Autodesk Inventor part; units mm, degrees
ref_plane "Плоскость YZ" through (0, 0, 0) normal (1, 0, 0) x (0, 1, 0)
ref_plane "Плоскость XZ" through (0, 0, 0) normal (0, 1, 0) x (-1, 0, 0)
ref_plane "Плоскость XY" through (0, 0, 0) normal (0, 0, 1) x (1, 0, 0)
sketch "Эскиз1" plane through (0, 0, 0) normal (0, 1, 0) x (-1, 0, 0)
  line L0 (9.1667, 12.5) -> (-9.1667, 12.5)
  line L1 (-9.1667, 12.5) -> (-9.1667, -12.5)
  line L2 (-9.1667, -12.5) -> (9.1667, -12.5)
  line L3 (9.1667, -12.5) -> (9.1667, 12.5)
  line L4 (9.1667, 12.5) -> (-9.1667, -12.5) construction
  line L5 (-9.1667, 12.5) -> (9.1667, -12.5) construction
  line L6 (10.7667, 14.5) -> (-10.7667, 14.5)
  line L7 (-10.7667, 14.5) -> (-10.7667, -14.5)
  line L8 (-10.7667, -14.5) -> (10.7667, -14.5)
  line L9 (10.7667, -14.5) -> (10.7667, 14.5)
  line L10 (10.7667, 14.5) -> (-10.7667, -14.5) construction
  line L11 (-10.7667, 14.5) -> (10.7667, -14.5) construction
  circle A0 centre (6.6667, 10) radius 1.5
  circle A1 centre (6.6667, 3.3333) radius 1.5
  circle A2 centre (6.6667, -3.3333) radius 1.5
  circle A3 centre (6.6667, -10) radius 1.5
  circle A4 centre (0, 10) radius 1.5
  circle A5 centre (0, 3.3333) radius 1.5
  circle A6 centre (0, -3.3333) radius 1.5
  circle A7 centre (0, -10) radius 1.5
  circle A8 centre (-6.6667, 10) radius 1.5
  circle A9 centre (-6.6667, 3.3333) radius 1.5
  circle A10 centre (-6.6667, -3.3333) radius 1.5
  circle A11 centre (-6.6667, -10) radius 1.5
  point P0 (0, 0)
  dimension "d0" = 18.3333
  dimension "d1" = 25
  dimension "d2" = 1.6
  dimension "d3" = 2
  dimension "d4" = 3
  dimension "d5" = 2.5
  dimension "d6" = 2.5
  dimension "d9" = 6.6667
  dimension "d12" = 6.6667
extrude "Выдавливание1" add sketch "Эскиз1" along normal blind 1.8 contours L3 L2 L1 L0 | L9 L8 L7 L6
sketch "Эскиз2" plane through (0, 1.8, 0) normal (0, 1, 0) x (1, 0, 0)
  circle A0 centre (6.6667, 10) radius 1.5
  circle A1 centre (6.6667, -3.3333) radius 1.5
  circle A2 centre (0, 10) radius 1.5
  circle A3 centre (0, 3.3333) radius 1.5
  circle A4 centre (0, -3.3333) radius 1.5
  circle A5 centre (0, -10) radius 1.5
  circle A6 centre (-6.6667, 10) radius 1.5
  circle A7 centre (-6.6667, 3.3333) radius 1.5
  circle A8 centre (-6.6667, -3.3333) radius 1.5
  circle A9 centre (-6.6667, -10) radius 1.5
  circle A10 centre (6.6667, -10) radius 1.5
  circle A11 centre (6.6667, 3.3333) radius 1.5
  circle A12 centre (6.6667, 10) radius 1.5
  circle A13 centre (6.6667, 10) radius 2.8
  point P0 (0, 0)
  dimension "d39" = 5.6
extrude "Выдавливание2" cut sketch "Эскиз2" against normal blind 0.7 contours A13
sketch "Эскиз3" plane through (0, 1.8, 0) normal (0, 1, 0) x (1, 0, 0)
  line L0 (-10.7667, 14.5) -> (-10.7667, -14.5)
  line L1 (10.7667, 14.5) -> (-10.7667, 14.5)
  line L2 (-10.7667, -14.5) -> (-9.9667, -14.5)
  line L3 (-9.9667, -14.5) -> (-9.9667, 14.5)
  line L4 (-9.9667, 14.5) -> (-10.7667, 14.5)
  line L5 (-10.7667, 14.5) -> (-10.7667, -14.5)
  line L6 (10.7667, -14.5) -> (10.7667, 14.5)
  line L7 (10.7667, -14.5) -> (9.9667, -14.5)
  line L8 (9.9667, -14.5) -> (9.9667, 14.5)
  line L9 (9.9667, 14.5) -> (10.7667, 14.5)
  line L10 (10.7667, 14.5) -> (10.7667, -14.5)
  point P0 (0, 0)
  point P1 (9.9667, 14.5)
  dimension "d29" = 0.8
  dimension "d30" = 0.8
extrude "Выдавливание3" add sketch "Эскиз3" along normal blind 1.2
pattern_linear "Прямоуг.массив2" count 4 spacing 6.6667 along (0, 0, 1) count 3 spacing 6.6667 along (-1, 0, 0) of "Выдавливание2"
equation "\"d6\" = d5"
equation "\"d30\" = d29"
properties part number "HolesHelper" material "Типовой"
Design review of the part built by this model. Coordinates are the model's own, in mm. A direction names the side the tool comes from. Coordinates: 2 decimals unless noted, no trailing zeros. Order: outer loops, then holes, each group sorted by start corner. A loop starts at its lowest first (then second) coordinate and runs counter-clockwise, first axis right, second up. Notation, with made-up numbers: M 41,-14.5 L 67,-14.5 A11 ccw 67,-10.5 Z; hole C 31.25,51.25 d11. An arc over 180 degrees is marked long. Use a Markdown table: item, result.
(1) Add section B-B (z = -10). Count the separate pieces of the cut face and the enclosed holes in it, then the cut area to 3 significant figures.
Worked answers:
| item | result |
|---|---|
| separate pieces | 4 |
| enclosed holes | 0 |
| area | 19.0 mm2 |
(2) Add section A-A (y = 2.1). Give the boundary of the cut face in (x, z).
Worked answers:
| item | result |
|---|---|
| outline | M -10.77,-14.5 L -9.97,-14.5 L -9.97,14.5 L -10.77,14.5 Z; M 9.97,-14.5 L 10.77,-14.5 L 10.77,14.5 L 9.97,14.5 Z |
(3) For faces 1 (the cylindrical face through (-5.17, 0.54, -3.4)), 2 (the cylindrical face through (-3.996, 1.455, -4.174)), list the 3-axis set-ups (+Z, -Z, +X, -X, +Y, -Y) from which the entire face can be reached by the end or side of a thin tool; tool diameter is ignored.
Worked answers:
| item | result |
|---|---|
| face 1 | +Y, -Y |
| face 2 | +Y |
(4) Wall thickness on probe 1 along Z at (x, y) = (0, 0.9); probe 2 along Z at (x, y) = (0, 1.35); probe 3 along X at (y, z) = (1.55, -2.5): over which ranges is each line inside the solid? List them lowest first.
Worked answers:
| item | result |
|---|---|
| probe 1 | z = -14.5 to -11.5, -8.5 to -4.83, -1.83 to 1.83, 4.83 to 8.5, 11.5 to 14.5 |
| probe 2 | z = -14.5 to -12.8, -7.2 to -6.13, -0.53 to 0.53, 6.13 to 7.2, 12.8 to 14.5 |
| probe 3 | x = -10.77 to -9.34, -3.99 to -2.67, 2.67 to 3.99, 9.34 to 10.77 |
(5) For P1, Ø1.8, axis at x = 6.67, z = 10, coming from the -Y side; P2, Ø5, axis at x = -6.67, z = -10, coming from the +Y side; P3, Ø10, axis at x = -3.5, z = -3.5, coming from the +Y side; P4, Ø7.5, axis at x = -6.67, z = 3.33, coming from the +Y side, all flat-tipped, find the tip position at first contact; note any pin that passes through.
Worked answers:
| item | result |
|---|---|
| P1 | passes through |
| P2 | stops at y = 1.1 |
| P3 | stops at y = 1.8 |
| P4 | stops at y = 3 |
(6) Draft analysis for pull direction X (two halves, no side actions). For faces 3 (the cylindrical face through (-2.064, 1.455, -11.892)), 4 (the flat face through (-10.767, 1, 0)), 5 (the flat face through (0, 0, 0)), state which applies: released by +X, released by -X, zero draft, split by the parting line, or undercut.
Worked answers:
| item | result |
|---|---|
| face 3 | undercut |
| face 4 | released by -X |
| face 5 | zero draft |
